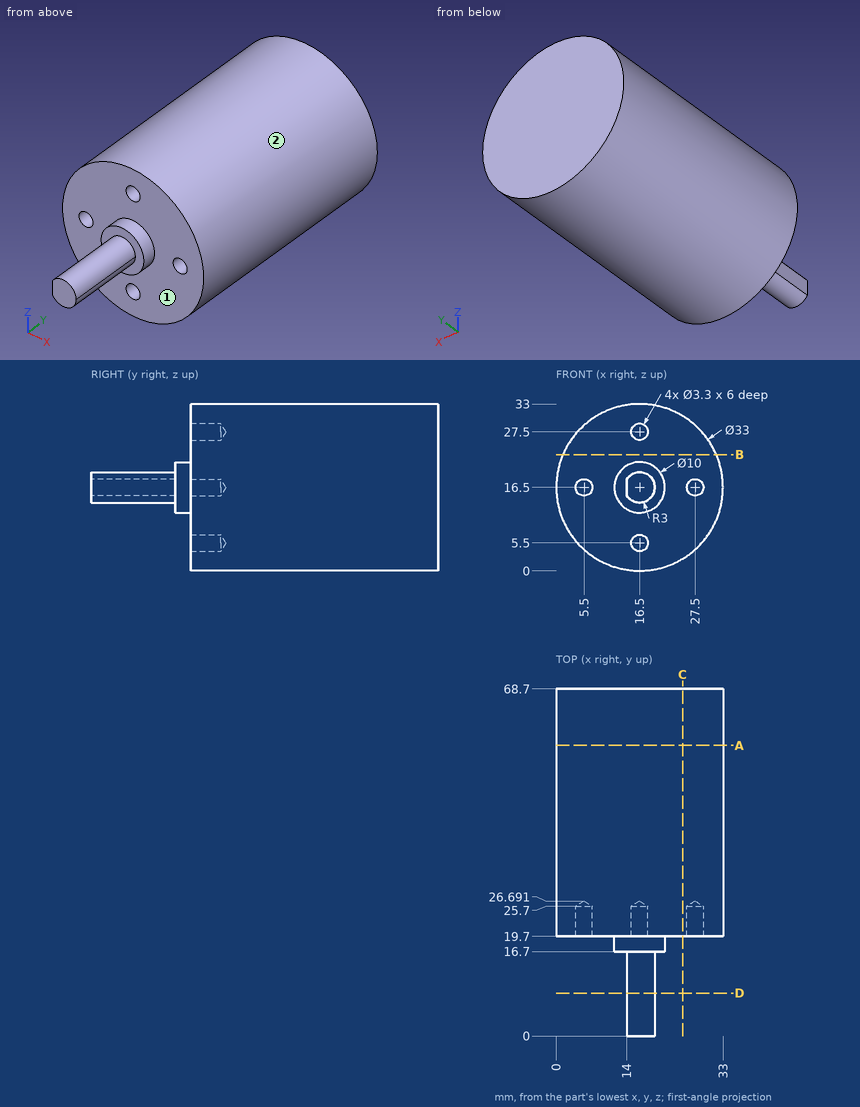
Could you check a few things on this drawing? It's one solid part, dimensions in mm from its lowest x, y, z. A direction names the side the tool comes from. Give positions to 0.01 mm unless a question says otherwise; leave off trailing zeros. Order: outer loops, then holes, each group sorted by start corner. A loop starts at its lowest first (then second) coordinate and runs counter-clockwise, first axis right, second up. Notation, with made-up numbers: (25, 54.5) - (55, 54.5) arc R9 ccw to (55, 66.5) - close; hole circle Ø9 at (-15.5, 74). An arc over 180 degrees is marked (long way). Return JSON: item names as keys, results as strings. Group by question number.
Q1. Suppose I cut it at A-A, the plane y = 57.5. Please give me the cut outline in (x, z).
Q2. Please list where these lines run through material, in increasing order: line 1 along Z through (x, y) = (16.5, 23.1); line 2 along Y through (x, z) = (10.5, 28.5); line 3 along Y through (x, z) = (12, 16). Write a range as [from, to].
Q3. Which directions (+Z, -Z, +X, -X, +Y, -Y) give clear straight access to the entire face, cutting with the end or side of a thin tool? Please do the marked faces 1 and 2.
Q4. Suppose I cut it at C-C, the plane x = 25. Please give me the cut outline in (y, z), and give its area (3 significant figures).
Q5. Will these pins go through, and if not, where does the flat tip stop? pin 1 Ø1.5 at (x, y) = (3.5, 61) entering from +Z (1 decimal); pin 2 Ø3.5 at (y, z) = (6, 16) entering from -X; pin 3 Ø4 at (y, z) = (18, 25) entering from +X (1 decimal); pin 4 Ø3 at (x, y) = (24.5, 17) entering from +Z.
Q6. Suppose I cut it at B-B, the plane z = 23. Please give me the cut outline in (x, y) (1 decimal), and give its area (3 significant figures).
Q7. Suppose I cut it at D-D, the plane y = 8.5. Please give me the cut outline in (x, z).
Resolved:
{
 "1": {"outline": "circle Ø33 at (16.5, 16.5)"},
 "2": {"line 1": "z = [0, 3.85], [7.15, 25.85], [29.15, 33]", "line 2": "y = [19.7, 68.7]", "line 3": "y = [16.7, 68.7]"},
 "3": {"face 1": "-Y", "face 2": "+Y, -Y"},
 "4": {"outline": "(19.7, 2.36) - (68.7, 2.36) - (68.7, 30.64) - (19.7, 30.64) - close", "area": "1,390 mm2"},
 "5": {"pin 1": "stops at z = 27.6", "pin 2": "stops at x = 14", "pin 3": "stops at x = 31.2", "pin 4": "passes through"},
 "6": {"outline": "(1.3, 19.7) - (31.7, 19.7) - (31.7, 68.7) - (1.3, 68.7) - close", "area": "1,490 mm2"},
 "7": {"outline": "(14, 14.84) arc R3 ccw (long way) to (14, 18.16) - close"}
}
